Geometry check sheet. Reference: the model listing, model coordinates, mm. A direction names the side the tool comes from. Round coordinates to 2 decimals unless told otherwise and drop trailing zeros. Write each loop counter-clockwise with the first axis right and the second up, starting at its lowest first coordinate (ties: lowest second). Pieces come first, ordered by that corner, then holes.
Item 1: Access from +Z, -Z, +X, -X, +Y, -Y to the whole of each face (thin tool, end or side, straight path). Record for faces 1 (the face through (0, 107, 22.5)), 2 (the face through (-0.11, 117.73, -0.5)), 3 (the face through (0, 107, -22.5)), 4 (the face through (20, 92.5, 11)).
Item 2: Cross-section at D-D (y = 86). Enter the section's corners in (x, z).
Item 3: Scan lines: probe 1 along Y at (x, z) = (9, 22.5); probe 2 along Y at (x, z) = (-14, -15); probe 3 along X at (y, z) = (33, 1). Record each from-to range of solid material in increasing order.
Item 4: Depth check by flat-ended pin: P1, Ø8, axis at y = 125.5, z = -0.5, coming from the -X side; P2, Ø10, axis at y = 82.5, z = -7, coming from the +X side; P3, Ø16.5, axis at x = 2.5, y = 109.5, coming from the -Z side; P4, Ø22, axis at x = 2.5, z = -3.5, coming from the -Y side. Enter the tip coordinate at first touch or a pass-through.
Item 5: Draft check along X on faces 5 (the face through (-7.5, 118, -5)), 6 (the face through (7.5, 118, -5)), 7 (the face through (-2.17, 36.98, -9.76)), 8 (the face through (13, 100, 0)). Enter one of: pulls with the +X half, pulls with the -X half, needs draft (parallel to the pull), parting line crosses it, or undercut.
Item 6: Cross-section at B-B (y = 129.5). Enter the section's corners in (x, z).
Item 7: Cross-section at C-C (x = -20). Enter the section's corners in (y, z), then the cut area to 3 significant figures.
Item 8: Cross-section at A-A (z = 8). Enter the section's corners in (x, y).
Autodesk Inventor part; units mm, degrees
ref_plane "YZ Plane" through (0, 0, 0) normal (1, 0, 0) x (0, 1, 0)
ref_plane "XZ Plane" through (0, 0, 0) normal (0, 1, 0) x (-1, 0, 0)
ref_plane "XY Plane" through (0, 0, 0) normal (0, 0, 1) x (1, 0, 0)
sketch "Sketch1" plane through (0, 0, 0) normal (1, 0, 0) x (0, 1, 0)
  line L0 (0, 0) -> (100, 0)
  line L1 (100, 0) -> (100, -30)
  line L2 (100, -30) -> (92.5, -30)
  line L3 (92.5, -30) -> (92.5, -22.4)
  line L4 (92.5, -22.4) -> (0, -22.4)
  line L5 (0, -22.4) -> (0, 0)
  line L6 (100, 0) -> (100, -22.5)
  line L7 (100, -22.5) -> (115, -22.5)
  line L8 (100, 0) -> (100, 22.5)
  line L9 (100, 22.5) -> (115, 22.5)
  circle A0 centre (127.721, -0.0575) radius 10
  arc A1 (146.8198, 0) -> (115, 22.5) centre (115, -11.25) ccw
  arc A2 (115, -22.5) -> (146.8198, 0) centre (115, 11.25) ccw
  dimension "d0" = 100
  dimension "d1" = 30
  dimension "d2" = 7.5
  dimension "d3" = 7.6
  dimension "d9" = 22.5
  dimension "d10" = 15
  dimension "d11" = 22.5
  dimension "d15" = 20
  dimension "d26" = 33.75
  dimension "d27" = 33.75
revolve "Revolution1" add sketch "Sketch1" angle 360 about axis through (0, 0, 0) along (0, 1, 0) contours L0 L1 L2 L3 L4 L5
extrude "Extrusion1" add sketch "Sketch1" along normal mid plane 15 contours L8 L9 A1 A2 L7 L1
fillet "Fillet1" radius 5 1 edges at (0, 146.8198, 0)
thread "Thread1"
sketch "Sketch2" plane through (0, 0, 0) normal (0, -1, 0) x (1, 0, 0)
  circle A0 centre (0, 0) radius 10
  dimension "d23" = 20
extrude "Extrusion2" cut sketch "Sketch2" against normal blind 75
properties material "Aluminum 6061"
Resolved:
1. face 1: +Z, +X, -X, +Y
1. face 2: +X, -X
1. face 3: -Z, +X, -X, +Y
1. face 4: -Y
2. outline: circle Ø44.8 at (0, 0)
3. probe 1: y = 92.5 to 100
3. probe 2: y = 0 to 100
3. probe 3: x = -22.38 to -9.95, 9.95 to 22.38
4. P1: passes through
4. P2: stops at x = 22.31
4. P3: stops at z = -22.5
4. P4: stops at y = 0
5. face 5: pulls with the -X half
5. face 6: pulls with the +X half
5. face 7: undercut
5. face 8: needs draft
6. outline: (-7.5, -19.23) - (7.5, -19.23) - (7.5, -9.9) - (-7.5, -9.9) - close; (-7.5, 9.78) - (7.5, 9.78) - (7.5, 19.23) - (-7.5, 19.23) - close
7. outline: (0, -10.09) - (92.5, -10.09) - (92.5, -22.36) - (100, -22.36) - (100, 22.36) - (92.5, 22.36) - (92.5, 10.09) - (0, 10.09) - close
7. area: 2,200 mm2
8. outline: (-28.91, 92.5) - (-20.92, 92.5) - (-20.92, 0) - (-6, 0) - (-6, 75) - (6, 75) - (6, 0) - (20.92, 0) - (20.92, 92.5) - (28.91, 92.5) - (28.91, 100) - (7.5, 100) - (7.5, 121.8) - (-7.5, 121.8) - (-7.5, 100) - (-28.91, 100) - close; (-7.5, 133.64) - (7.5, 133.64) - (7.5, 142.72) - (-7.5, 142.72) - close
